```python
from build123d import *

# Parameters (mm, degrees)
SKETCH_W        = 53
SKETCH_H        = 29
PAD_DEPTH       = 40.45
SKETCH001_W     = 29
SKETCH001_H     = 6.6
SKETCH001_H_2   = 27.45
POCKET_DEPTH    = 7.5
SKETCH002_R     = 1
POCKET001_DEPTH = 6.5
PAD001_DEPTH    = 2.5
SKETCH004_W     = 45
SKETCH004_H     = 2
PAD002_DEPTH    = 6.6


with BuildPart() as part:
    # Sketch → Pad (new body)
    with BuildSketch(Plane.XY):
        with Locations((-26.5, 0)):
            Rectangle(SKETCH_W, SKETCH_H)
    extrude(amount=PAD_DEPTH)

    # Sketch001 → Pocket (cut)
    with BuildSketch(Plane.YZ):
        with Locations((0, 37.15)):
            Rectangle(SKETCH001_W, SKETCH001_H)
        with Locations((0, 13.725)):
            Rectangle(SKETCH001_W, SKETCH001_H_2)
    extrude(amount=-POCKET_DEPTH, mode=Mode.SUBTRACT)

    # Sketch002 → Pocket001 (cut)
    with BuildSketch(Plane.XY.offset(33.85)):
        with Locations((-3, -11.5)):
            Circle(SKETCH002_R)
        with Locations((-3, 11.5)):
            Circle(SKETCH002_R)
        with BuildLine():
            Line((-3, 8.5), (-7.5, 8.5))
            Line((-7.5, 8.5), (-7.5, -8.5))
            Line((-7.5, -8.5), (-3, -8.5))
            ThreePointArc((-3, -14.5), (0, -11.5), (-3, -8.5))
            Line((-3, -14.5), (2, -14.5))
            Line((2, -14.5), (2, 14.5))
            Line((2, 14.5), (-3, 14.5))
            ThreePointArc((-3, 8.5), (0, 11.5), (-3, 14.5))
        make_face()
    extrude(amount=-POCKET001_DEPTH, mode=Mode.SUBTRACT)

    # Sketch003 → Pad001 (new body)
    with BuildSketch(Plane.YZ.offset(-7.5)):
        with BuildLine():
            Line((-21.896552, 10.541379), (-15, 3.3))
            Line((-15, 3.3), (15, 3.3))
            Line((15, 3.3), (21.896552, 10.541379))
            ThreePointArc((21.896552, 10.541379), (22.201473, 15.698034), (17.167124, 16.855357))
            Line((9, 13.3), (17.167124, 16.855357))
            Line((-9, 13.3), (9, 13.3))
            Line((-17.167124, 16.855357), (-9, 13.3))
            ThreePointArc((-17.167124, 16.855357), (-22.201473, 15.698034), (-21.896552, 10.541379))
        make_face()
    extrude(amount=PAD001_DEPTH)

    # Sketch004 → Pad002 (new body)
    with BuildSketch(Plane.YZ.offset(-7.5)):
        with Locations((0, 1)):
            Rectangle(SKETCH004_W, SKETCH004_H)
    extrude(amount=PAD002_DEPTH)


solid = part.part
```
The listing builds one solid part. Answer for the finished solid, in the listing's coordinates (mm). A direction names the side the tool comes from. Coordinates: 2 decimals unless noted, no trailing zeros. Write each loop counter-clockwise with the first axis right and the second up, starting at its lowest first coordinate (ties: lowest second). Pieces come first, ordered by that corner, then holes. Notation, with made-up numbers: M 26,51 L 80,51 A15 ccw 80,71 Z; hole C -40,77.5 d2. An arc over 180 degrees is marked long. Use a Markdown table: item, result. Add a question column.
1. Section D-D (y = 0) is taken. Give the vertices of the cut face in (x, z).
2. Straight lines are drawn through the part: line 1 along Y through (x, z) = (-3, 29); line 2 along X through (y, z) = (14, 24.5); line 3 along Y through (x, z) = (-49, 18.5). For each, find the intervals that lie inside material, in ascending order. Write a range as [from, to].
3. Section C-C (x = -12.5) is taken. Give the vertices of the cut face in (y, z).
4. Which of the six approach directions +Z, -Z, +X, -X, +Y, -Y give full straight-line access (tool end or side, diameter ignored) to faces 4 (the flat face through (-7.5, -18, 12)), 5 (the flat face through (-4, -22.5, 1)), 6 (the cylindrical face through (0, -11.6, 30.7)), 7 (the flat face through (-6, 0, 3.3))?
5. Section B-B (z = 22) is taken. Give the vertices of the cut face in (x, y), plus the area to 3 significant figures.
6. Given P1, Ø2.5, axis at x = -3, y = 11.5, coming from the +Z side; P2, Ø4, axis at x = -33, z = 9, coming from the +Y side; P3, Ø4, axis at y = -3, z = 7.5, coming from the +X side, each flat-ended and moving along its own axis, determine where each tip first touches the part or whether it passes through.
7. For a pull along Y with two mould halves and no side action, classify faces 1 (the flat face through (-5, -12, 33.85)), 2 (the flat face through (-6.27, 18.4, 6.87)), 3 (the flat face through (-5, -8.5, 31)) as +Y half, -Y half, draft (parallel to the pull), parting line (faces both ways), or undercut.
8. Section A-A (y = 11.5) is taken. Give the vertices of the cut face in (x, z).
Data:
| question | item | result |
|---|---|---|
| 1 | outline | M -53,0 L -0.9,0 L -0.9,2 L -7.5,2 L -7.5,3.3 L -5,3.3 L -5,13.3 L -7.5,13.3 L -7.5,40.45 L -53,40.45 Z |
| 2 | line 1 | y = [-14.5, -12.5], [-10.5, -8.5], [8.5, 10.5], [12.5, 14.5] |
| 2 | line 2 | x = [-53, -7.5] |
| 2 | line 3 | y = [-14.5, 14.5] |
| 3 | outline | M -14.5,0 L 14.5,0 L 14.5,40.45 L -14.5,40.45 Z |
| 4 | face 4 | +Z, -Z, -X, -Y |
| 4 | face 5 | -Z, +X, -X, -Y |
| 4 | face 6 | +Z, +X |
| 4 | face 7 | +X, +Y, -Y |
| 5 | outline | M -53,-14.5 L -7.5,-14.5 L -7.5,14.5 L -53,14.5 Z |
| 5 | area | 1,320 mm2 |
| 6 | P1 | stops at z = 33.85 |
| 6 | P2 | stops at y = 14.5 |
| 6 | P3 | stops at x = -5 |
| 7 | face 1 | draft |
| 7 | face 2 | +Y half |
| 7 | face 3 | undercut |
| 8 | outline | M -53,0 L -0.9,0 L -0.9,2 L -7.5,2 L -7.5,3.3 L -5,3.3 L -5,14.39 L -7.5,14.39 L -7.5,27.45 L -4,27.45 L -4,33.85 L -7.5,33.85 L -7.5,40.45 L -53,40.45 Z; M -2,27.45 L 0,27.45 L 0,33.85 L -2,33.85 Z |
